Autodesk Fusion 360 part; units mm, degrees
sketch "Sketch1" plane through (0, 0, 0) normal (0, 0, 1) x (1, 0, 0)
  line L0 (-5, 0) -> (-5, -50)
  line L1 (5, 0) -> (5, -50)
  line L2 (5, 0) -> (45, 0)
  line L3 (-5, 0) -> (-45, 0)
  line L4 (5, -50) -> (45, -50)
  line L5 (-5, -50) -> (-45, -50)
  line L6 (70, -25) -> (70.7973, -25) construction
  circle A0 centre (-45, -25) radius 12.5
  circle A1 centre (45, -25) radius 12.5
  arc A2 (-45, 0) -> (-45, -50) centre (-45, -25) ccw
  arc A3 (45, -50) -> (45, 0) centre (45, -25) ccw
  line L7 (-5, 0) -> (5, 0)
  line L8 (-5, -50) -> (5, -50)
  dimension "d4" = 40
  dimension "d5" = 40
  dimension "d6" = 40
  dimension "d7" = 40
  dimension "d8" = 25
  dimension "d9" = 50
  dimension "d10" = 25
  dimension "d11" = 50
extrude "Extrude1" add sketch "Sketch1" along normal blind 10 contours L0 L3 L5 A2 | L1 L2 L4 A3 makes body 1 at (-14.1667, -25, 0) makes body 2 at (14.1667, -25, 0)
extrude "Extrude2" add sketch "Sketch1" along normal blind 50 contours L0 L1 L7 L8 bodies 1 2
sketch "Sketch2" plane through (5, 0, 0) normal (1, 0, 0) x (0, 1, 0)
  line L0 (-50, 10) -> (0, 10)
  line L1 (0, 10) -> (0, 50)
  line L2 (0, 50) -> (-50, 50)
  line L3 (-50, 50) -> (-50, 10)
  arc A0 (0, 50) -> (-50, 50) centre (-25, 50) ccw
  circle A1 centre (-25, 50) radius 12.5
  dimension "d16" = 50
  dimension "d17" = 25
extrude "Extrude3" add sketch "Sketch2" against normal blind 10 contours L2 A0 A1 bodies 1
hole "Hole1" at (5, -25, 50) direction (-1, 0, 0) diameter 30 depth 30 tip angle 118 bodies 1
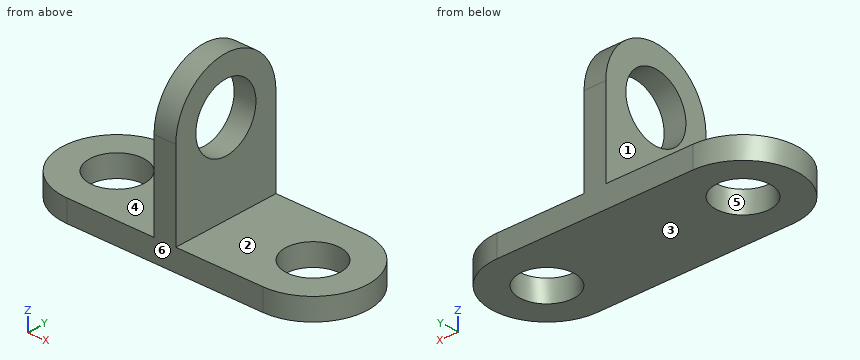
The model under review builds one solid part; all positions refer to its coordinate system, in mm. Face numbers are marked on the shaded views. A direction names the side the tool comes from. Give positions to 0.01 mm unless a question says otherwise; leave off trailing zeros. Order: outer loops, then holes, each group sorted by start corner. A loop starts at its lowest first (then second) coordinate and runs counter-clockwise, first axis right, second up. Notation, with made-up numbers: M -34.75,-29.5 L 13.25,-29.5 A5 ccw 13.25,-25.5 Z; hole C 6,34.5 d8. An arc over 180 degrees is marked long. Use one line per item in the form item = value. Start each with the question number.
Item 1: For the marked faces 1, 2 and 3, list the 3-axis set-ups (+Z, -Z, +X, -X, +Y, -Y) from which the entire face can be reached by the end or side of a thin tool; tool diameter is ignored.
Item 2: Insertion check: pin 1 Ø3 at (y, z) = (-5.5, 63) entering from +X; pin 2 Ø25 at (y, z) = (-27, 58.5) entering from -X; pin 3 Ø1 at (x, y) = (-0.5, -25.5) entering from +Z. Each pin has a flat end and moves straight along its axis. Give the tip position at first contact, or say it passes through.
Item 3: We need section D-D on z = 20. Give the boundary of the cut face in (x, y), plus the area to 3 significant figures.
Item 4: To check wall thickness, follow line 1 along Y through (x, z) = (45, 3); line 2 along Y through (x, z) = (0.5, 50); line 3 along Z through (x, y) = (-2.5, -25). State the ranges of each line that lie inside material, in increasing order. Write a range as from..to.
Item 5: We need section C-C on y = -7. Give the boundary of the cut face in (x, z), plus the area to 3 significant figures.
Item 6: We need section A-A on y = -25. Give the boundary of the cut face in (x, z).
Item 7: The part is to be moulded in two halves that separate along Y. For the marked faces 4, 5 and 6, say which applies: pulls with the +Y half, pulls with the -Y half, needs draft (parallel to the pull), parting line crosses it, or undercut.
Item 8: We need section B-B on x = 47. Give the boundary of the cut face in (y, z), plus the area to 3 significant figures.
Completed:
q1.face_1 = +Z, -X, +Y, -Y
q1.face_2 = +Z, +X, +Y, -Y
q1.face_3 = -Z, +X, -X, +Y, -Y
q2.pin_1 = 5
q2.pin_2 = -5
q2.pin_3 = 75
q3.outline = M -5,-50 L 5,-50 L 5,0 L -5,0 Z
q3.area = 500 mm²
q4.line_1 = -50..-37.5, -12.5..0
q4.line_2 = -50..-40, -10..0
q4.line_3 = 0..35, 65..75
q5.outline = M -62.35,0 L 62.35,0 L 62.35,10 L 5,10 L 5,67.35 L -5,67.35 L -5,10 L -62.35,10 Z
q5.area = 1,820 mm²
q6.outline = M -70,0 L -57.5,0 L -57.5,10 L -70,10 Z; M -32.5,0 L 32.5,0 L 32.5,10 L 5,10 L 5,35 L -5,35 L -5,10 L -32.5,10 Z; M -5,65 L 5,65 L 5,75 L -5,75 Z; M 57.5,0 L 70,0 L 70,10 L 57.5,10 Z
q7.face_4 = needs draft
q7.face_5 = undercut
q7.face_6 = pulls with the -Y half
q8.outline = M -49.92,0 L -37.34,0 L -37.34,10 L -49.92,10 Z; M -12.66,0 L -0.08,0 L -0.08,10 L -12.66,10 Z
q8.area = 252 mm²
